from build123d import *

# Parameters (mm, degrees)
F0_W     = 12.7
F0_H     = 7.747
F0_H_2   = 3.175
F0_W_2   = 3.175
F3_DEPTH = 15.876
F4_SIZE  = 0.254
F5_R     = 3.175
F6_DEPTH = 12.7


with BuildPart() as f1:
    # F0 (on Right) → F1 (revolve)
    with BuildSketch(Plane.YZ):
        with Locations((0, 7.0485)):
            Rectangle(F0_W, F0_H)
        with Locations((0, 1.5875)):
            Rectangle(F0_W, F0_H_2)
        with Locations((-7.9375, 1.5875)):
            Rectangle(F0_W_2, F0_H_2)
        with Locations((7.9375, 1.5875)):
            Rectangle(F0_W_2, F0_H_2)
    revolve(axis=Axis((0, 0, 0), (0, 1, 0)))

    # F2 (on face) → F3 (cut, through all)
    with BuildSketch(Plane.XZ.offset(6.35)):
        with BuildLine():
            Line((-8.9757648699, -6.223), (-10.8736076074, -6.223))
            Line((-10.8736076074, -6.223), (-10.8736076074, -16.0401048288))
            Line((-10.8736076074, -16.0401048288), (15.6559471654, -16.0401048288))
            Line((15.6559471654, -16.0401048288), (15.6559471654, -6.223))
            Line((15.6559471654, -6.223), (8.9757648699, -6.223))
            ThreePointArc((8.9757648699, -6.223), (0, -10.922), (-8.9757648699, -6.223))
        make_face()
        with BuildLine():
            Line((8.9757648699, -6.223), (-8.9757648699, -6.223))
            ThreePointArc((-8.9757648699, -6.223), (0, -10.922), (8.9757648699, -6.223))
        make_face()
    extrude(amount=-F3_DEPTH, mode=Mode.SUBTRACT)

    # F4
    f4_edges = [f1.edges().sort_by_distance(p)[0] for p in [
        (0, -9.525, -3.175),
        (0, -6.35, 10.922),
        (0, 6.35, 10.922),
        (0, 9.525, -3.175),
    ]]
    chamfer(f4_edges, length=F4_SIZE)

    # F5 (on face) → F6 (cut)
    with BuildSketch(Plane(origin=(0, 0, -6.223), x_dir=(1, 0, 0), z_dir=(0, 0, -1))):
        Circle(F5_R)
    extrude(amount=-F6_DEPTH, mode=Mode.SUBTRACT)


solid = f1.part
Work out the finished part from the listing and answer in its coordinate system (mm). A direction names the side the tool comes from. Coordinates: 2 decimals unless noted, no trailing zeros. Write each loop counter-clockwise with the first axis right and the second up, starting at its lowest first coordinate (ties: lowest second). Pieces come first, ordered by that corner, then holes. Notation, with made-up numbers: M 51,-12.75 L 72,-12.75 A20 ccw 72,10.25 Z; hole C 19,-37 d2. An arc over 180 degrees is marked long. Use one line per item in the form item = value. Start each with the question number.
1. Each of these flat-tipped pins is pushed along its axis until it touches: P1, Ø2, axis at y = 0.5, z = -2, coming from the +X side; P2, Ø4, axis at x = -7, z = 0.5, coming from the -Y side; P3, Ø2, axis at x = 6, z = -1.5, coming from the +Y side. Where does it stop, or does it pass through?
2. The part is cut by section A-A (z = 0). Give the vertices of the cut face in (x, y) (3 decimals), plus the area to 3 significant figures.
3. The part is cut by section C-C (x = 0). Give the vertices of the cut face in (y, z) (3 decimals), plus the area to 3 significant figures.
4. Straight lines are drawn through the part: probe 1 along Y at (x, z) = (0, 1.25) (3 decimals); probe 2 along Y at (x, z) = (6.75, 7); probe 3 along X at (y, z) = (0, -1.5) (1 decimal). For each, find the intervals that lie inside material, in ascending order. Write a range as from..to.
5. The part is cut by section B-B (y = 0). Give the vertices of the cut face in (x, z) (3 decimals).
6. The part is cut by section D-D (y = 6.75). Give the vertices of the cut face in (x, z) (3 decimals).
7. A tool of negligible diameter and unlimited length cuts with its end or side. For faces 1 (the face through (-0.333, 0.085, 10.917)), 2 (the face through (-0.69, 3.1, 0.04)), 3 (the face through (-3.1, -7.79, -0.69)), 4 (the face through (0, -9.525, 0)), 5 (the face through (-3.1, 7.83, -0.69)), from which of +Z, -Z, +X, -X, +Y, -Y can it reach the whole face along a straight path? Write none if from no direction.
8. The mould has two halves that part along Y. Classify faces 6 (the face through (0.332, -6.221, 10.792)), 7 (the face through (0, 0, 6.477)), 8 (the face through (0, 6.35, 4)), 9 (the face through (2, 3, -6.223)): released by +Y, released by -Y, zero draft, split by the parting line, or undercut.
Evaluation:
q1.P1 = 10.88
q1.P2 = -6.35
q1.P3 = 6.35
q2.outline = M -10.922,-6.096 L -10.668,-6.35 L -3.175,-6.35 L -3.175,-9.271 L -2.921,-9.525 L 2.921,-9.525 L 3.175,-9.271 L 3.175,-6.35 L 10.668,-6.35 L 10.922,-6.096 L 10.922,6.096 L 10.668,6.35 L 3.175,6.35 L 3.175,9.271 L 2.921,9.525 L -2.921,9.525 L -3.175,9.271 L -3.175,6.35 L -10.668,6.35 L -10.922,6.096 Z; hole C 0,0 d6.35
q2.area = 286 mm^2
q3.outline = M -9.525,-2.921 L -9.271,-3.175 L -6.35,-3.175 L -6.35,-6.223 L -3.175,-6.223 L -3.175,6.477 L 3.175,6.477 L 3.175,-6.223 L 6.35,-6.223 L 6.35,-3.175 L 9.271,-3.175 L 9.525,-2.921 L 9.525,2.921 L 9.271,3.175 L 6.35,3.175 L 6.35,10.668 L 6.096,10.922 L -6.096,10.922 L -6.35,10.668 L -6.35,3.175 L -9.271,3.175 L -9.525,2.921 Z
q3.area = 177 mm^2
q4.probe_1 = -9.525..-3.175, 3.175..9.525
q4.probe_2 = -6.35..6.35
q4.probe_3 = -10.8..-3.2, 3.2..10.8
q5.outline = M -8.976,-6.223 L -3.175,-6.223 L -3.175,6.477 L 3.175,6.477 L 3.175,-6.223 L 8.976,-6.223 A10.922 ccw long Z
q6.outline = C 0,0 d6.35
q7.face_1 = +Y, -Y
q7.face_2 = -Z
q7.face_3 = -Y
q7.face_4 = +Z, -Z, +X, -X, -Y
q7.face_5 = +Y
q8.face_6 = released by -Y
q8.face_7 = undercut
q8.face_8 = released by +Y
q8.face_9 = zero draft
